Read the model definition and answer for the solid it produces. Units are mm, in the model's axes. Round coordinates to 2 decimals unless told otherwise and drop trailing zeros. Write each loop counter-clockwise with the first axis right and the second up, starting at its lowest first coordinate (ties: lowest second). Pieces come first, ordered by that corner, then holes. Notation, with made-up numbers: (38.5, 77) - (50.5, 77) arc R18 ccw to (50.5, 99) - close; hole circle Ø7 at (-32, 73.5). An arc over 180 degrees is marked (long way). Use one line per item in the form item = value. Start each with the question number.
1) The part is cut by section A-A, the plane y = 8.25. Give the vertices of the cut face in (x, z), plus the area to 3 significant figures.
2) Each of these flat-tipped pins is pushed along its axis until it touches: pin 1 (0.9 mm diameter, centred on y = 0.5, z = 2, fed in from -X); pin 2 (0.7 mm diameter, centred on y = 0.5, z = 0.5, fed in from -X); pin 3 (4 mm diameter, centred on x = 41.5, y = 7, fed in from +Z). Where does it stop, or does it pass through?
3) The part is cut by section B-B, the plane x = 7.5. Give the vertices of the cut face in (y, z), plus the area to 3 significant figures.
4) Consider line 1 along Z through (x, y) = (28, 7); line 2 along Y through (x, z) = (48, -0.1). Determine where each line is inside the solid, lowest interval first. Write a range as from..to.
from build123d import *

# Parameters (mm, degrees)
SKETCH_1_W                      = 90
SKETCH_1_H                      = 30
EXTRUDE_1_DEPTH                 = 2
SKETCH_2_W                      = 3
SKETCH_2_H                      = 3
EXTRUDE_2_DEPTH                 = 1
EXTRUDE_3_DEPTH                 = 2
CUT_EXTRUDE_1_REACH             = 87.55
CUT_EXTRUDE_1_DIRECTION_2_REACH = 87.55
FILLET_1_R                      = 0.1
FILLET_1_OF_MIRROR_1_R          = 0.1
FILLET_1_OF_MIRROR_3_R          = 0.1
FILLET_2_R                      = 0.2


# Read off the part's stored shape, not the designer's step: the mirror step
with BuildPart() as part:
    # Sketch 1 → Extrude 1 (new body)
    with BuildSketch(Plane.XY):
        with Locations((37.5, 7.5)):
            Rectangle(SKETCH_1_W, SKETCH_1_H)
    extrude(amount=-EXTRUDE_1_DEPTH)

    # Sketch 2 → Extrude 2 (add)
    with BuildSketch(Plane.XY):
        Rectangle(SKETCH_2_W, SKETCH_2_H)
    extrude_2 = extrude(amount=EXTRUDE_2_DEPTH)

    # Sketch 3 → Extrude 3 (add, symmetric)
    with BuildSketch(Plane(origin=(0, 0, 0), x_dir=(1, 0, 0), z_dir=(0, 1, 0))):
        with BuildLine():
            Line((-1.95, -2.5), (1.95, -2.5))
            Line((1.95, -2.5), (1.95, -1.555590279))
            ThreePointArc((1.95, -1.555590279), (1.780042303, -1.088161527), (1.5, -0.677124344))
            Line((1.5, -0.677124344), (-1.5, -0.677124344))
            ThreePointArc((-1.5, -0.677124344), (-1.780042303, -1.088161527), (-1.95, -1.555590279))
            Line((-1.95, -1.555590279), (-1.95, -2.5))
        make_face()
    extrude_3 = extrude(amount=EXTRUDE_3_DEPTH, both=True)

    # Sketch 4 → Cut-Extrude 1 (cut, up to next)
    with BuildSketch(Plane(origin=(0, 0, 0), x_dir=(0, 0, -1), z_dir=(1, 0, 0)), mode=Mode.PRIVATE) as cut_extrude_1_sk1:
        with BuildLine():
            Line((-2.5, 1.95), (-1.555590279, 1.95))
            ThreePointArc((-1.555590279, 1.95), (-1.088161527, 1.780042303), (-0.677124344, 1.5))
            Line((-0.677124344, 1.5), (-0.677124344, 2))
            Line((-0.677124344, 2), (-2.5, 2))
            Line((-2.5, 2), (-2.5, 1.95))
        make_face()
    cut_extrude_1_tool1 = extrude(cut_extrude_1_sk1.sketch, amount=-CUT_EXTRUDE_1_REACH, mode=Mode.PRIVATE) & part.part
    # Sketch 4 → Cut-Extrude 1 (cut, up to next)
    with BuildSketch(Plane(origin=(0, 0, 0), x_dir=(0, 0, -1), z_dir=(1, 0, 0)), mode=Mode.PRIVATE) as cut_extrude_1_sk2:
        with BuildLine():
            Line((-2.5, -2), (-0.677124344, -2))
            Line((-0.677124344, -2), (-0.677124344, -1.5))
            ThreePointArc((-0.677124344, -1.5), (-1.088161527, -1.780042303), (-1.555590279, -1.95))
            Line((-1.555590279, -1.95), (-2.5, -1.95))
            Line((-2.5, -1.95), (-2.5, -2))
        make_face()
    cut_extrude_1_tool2 = extrude(cut_extrude_1_sk2.sketch, amount=-CUT_EXTRUDE_1_REACH, mode=Mode.PRIVATE) & part.part
    cut_extrude_1_1 = cut_extrude_1_tool1.solids().sort_by_distance((0, 1.873038, 1.175075))[0]
    add(cut_extrude_1_1, mode=Mode.SUBTRACT)
    cut_extrude_1_2 = cut_extrude_1_tool2.solids().sort_by_distance((0, -1.873038, 1.175075))[0]
    add(cut_extrude_1_2, mode=Mode.SUBTRACT)
    cut_extrude_1 = cut_extrude_1_1 + cut_extrude_1_2  # Cut-Extrude 1 as one shape, for the pattern or mirror that repeats it

    # Sketch 4 → Cut-Extrude 1 direction 2 (cut, up to next)
    with BuildSketch(Plane(origin=(0, 0, 0), x_dir=(0, 0, -1), z_dir=(1, 0, 0)), mode=Mode.PRIVATE) as cut_extrude_1_direction_2_sk1:
        with BuildLine():
            Line((-2.5, 1.95), (-1.555590279, 1.95))
            ThreePointArc((-1.555590279, 1.95), (-1.088161527, 1.780042303), (-0.677124344, 1.5))
            Line((-0.677124344, 1.5), (-0.677124344, 2))
            Line((-0.677124344, 2), (-2.5, 2))
            Line((-2.5, 2), (-2.5, 1.95))
        make_face()
    cut_extrude_1_direction_2_tool1 = extrude(cut_extrude_1_direction_2_sk1.sketch, amount=CUT_EXTRUDE_1_DIRECTION_2_REACH, mode=Mode.PRIVATE) & part.part
    # Sketch 4 → Cut-Extrude 1 direction 2 (cut, up to next)
    with BuildSketch(Plane(origin=(0, 0, 0), x_dir=(0, 0, -1), z_dir=(1, 0, 0)), mode=Mode.PRIVATE) as cut_extrude_1_direction_2_sk2:
        with BuildLine():
            Line((-2.5, -2), (-0.677124344, -2))
            Line((-0.677124344, -2), (-0.677124344, -1.5))
            ThreePointArc((-0.677124344, -1.5), (-1.088161527, -1.780042303), (-1.555590279, -1.95))
            Line((-1.555590279, -1.95), (-2.5, -1.95))
            Line((-2.5, -1.95), (-2.5, -2))
        make_face()
    cut_extrude_1_direction_2_tool2 = extrude(cut_extrude_1_direction_2_sk2.sketch, amount=CUT_EXTRUDE_1_DIRECTION_2_REACH, mode=Mode.PRIVATE) & part.part
    cut_extrude_1_direction_2_1 = cut_extrude_1_direction_2_tool1.solids().sort_by_distance((0, 1.873038, 1.175075))[0]
    add(cut_extrude_1_direction_2_1, mode=Mode.SUBTRACT)
    cut_extrude_1_direction_2_2 = cut_extrude_1_direction_2_tool2.solids().sort_by_distance((0, -1.873038, 1.175075))[0]
    add(cut_extrude_1_direction_2_2, mode=Mode.SUBTRACT)
    cut_extrude_1_direction_2 = cut_extrude_1_direction_2_1 + cut_extrude_1_direction_2_2  # Cut-Extrude 1 direction 2 as one shape, for the pattern or mirror that repeats it

    # Fillet 1
    fillet_1_edges = [part.edges().sort_by_distance(p)[0] for p in [
        (-1.95, 0, 2.5),
        (1.95, 0, 2.5),
        (0, -1.95, 2.5),
        (0, 1.95, 2.5),
    ]]
    fillet(fillet_1_edges, radius=FILLET_1_R)

    # Mirror 1: Extrude 2, Extrude 3, Cut-Extrude 1, Cut-Extrude 1 direction 2 across plane
    add(extrude_2.mirror(Plane(origin=(7.5, 0, 0), x_dir=(0, 0, 1), z_dir=(1, 0, 0))))
    add(extrude_3.mirror(Plane(origin=(7.5, 0, 0), x_dir=(0, 0, 1), z_dir=(1, 0, 0))))
    add(cut_extrude_1.mirror(Plane(origin=(7.5, 0, 0), x_dir=(0, 0, 1), z_dir=(1, 0, 0))), mode=Mode.SUBTRACT)
    add(cut_extrude_1_direction_2.mirror(Plane(origin=(7.5, 0, 0), x_dir=(0, 0, 1), z_dir=(1, 0, 0))), mode=Mode.SUBTRACT)

    # Fillet 1 of Mirror 1
    fillet_1_of_mirror_1_edges = [part.edges().sort_by_distance(p)[0] for p in [
        (16.95, 0, 2.5),
        (13.05, 0, 2.5),
        (15, -1.95, 2.5),
        (15, 1.95, 2.5),
    ]]
    fillet(fillet_1_of_mirror_1_edges, radius=FILLET_1_OF_MIRROR_1_R)

    # Mirror 3: Extrude 2, Extrude 3, Cut-Extrude 1, Cut-Extrude 1 direction 2 across plane
    add(extrude_2.mirror(Plane(origin=(15, 0, 0), x_dir=(0, 0, 1), z_dir=(1, 0, 0))))
    add(extrude_3.mirror(Plane(origin=(15, 0, 0), x_dir=(0, 0, 1), z_dir=(1, 0, 0))))
    add(cut_extrude_1.mirror(Plane(origin=(15, 0, 0), x_dir=(0, 0, 1), z_dir=(1, 0, 0))), mode=Mode.SUBTRACT)
    add(cut_extrude_1_direction_2.mirror(Plane(origin=(15, 0, 0), x_dir=(0, 0, 1), z_dir=(1, 0, 0))), mode=Mode.SUBTRACT)

    # Fillet 1 of Mirror 3
    fillet_1_of_mirror_3_edges = [part.edges().sort_by_distance(p)[0] for p in [
        (31.95, 0, 2.5),
        (28.05, 0, 2.5),
        (30, -1.95, 2.5),
        (30, 1.95, 2.5),
    ]]
    fillet(fillet_1_of_mirror_3_edges, radius=FILLET_1_OF_MIRROR_3_R)

    # Mirror 4: part across plane


with BuildPart() as part_1:
    add(part.part)
    add(part.part.mirror(Plane(origin=(37.5, 0, 0), x_dir=(0, 0, 1), z_dir=(1, 0, 0))))

    # Fillet 2
    fillet_2_edges = [part_1.edges().sort_by_distance(p)[0] for p in [
        (82.5, 7.5, -2),
        (37.5, 22.5, -2),
        (-7.5, 7.5, -2),
        (37.5, 22.5, 0),
        (82.5, 7.5, 0),
        (37.5, -7.5, 0),
        (-7.5, 7.5, 0),
        (37.5, -7.5, -2),
        (-7.5, 22.5, -1),
        (82.5, 22.5, -1),
        (82.5, -7.5, -1),
        (-7.5, -7.5, -1),
    ]]
    fillet(fillet_2_edges, radius=FILLET_2_R)


solid = part_1.part
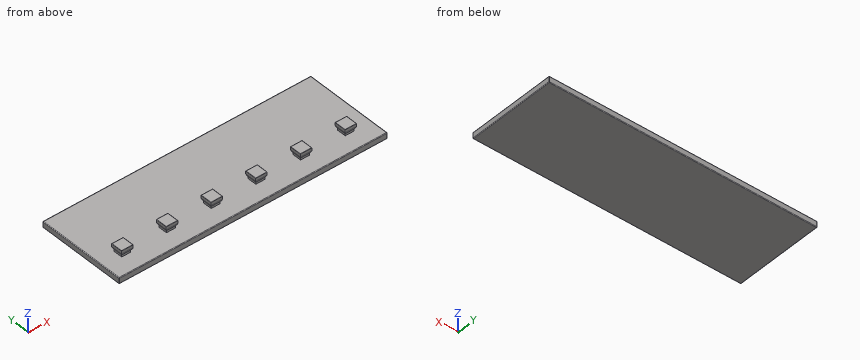
Geometry results:
q1.outline = (-7.5, -1.8) arc R0.2 ccw to (-7.3, -2) - (82.3, -2) arc R0.2 ccw to (82.5, -1.8) - (82.5, -0.2) arc R0.2 ccw to (82.3, 0) - (-7.3, 0) arc R0.2 ccw to (-7.5, -0.2) - close
q1.area = 180 mm2
q2.pin_1 = -1.95
q2.pin_2 = -1.64
q2.pin_3 = 0
q3.outline = (-7.5, -1.8) arc R0.2 ccw to (-7.3, -2) - (22.3, -2) arc R0.2 ccw to (22.5, -1.8) - (22.5, -0.2) arc R0.2 ccw to (22.3, 0) - (-7.3, 0) arc R0.2 ccw to (-7.5, -0.2) - close
q3.area = 60.0 mm2
q4.line_1 = -2..0
q4.line_2 = -7.47..22.47
